from build123d import *

# Parameters (mm, degrees)
SKETCH_1_R               = 45
EXTRUDE_2_DEPTH          = 19
SKETCH_3_R               = 30
EXTRUDE_3_DEPTH          = 34
SKETCH_8_R               = 23.5
CUT_EXTRUDE_2_DEPTH      = 14
SKETCH_9_R               = 31
CUT_EXTRUDE_4_DEPTH      = 14
SKETCH_11_R              = 25
CUT_EXTRUDE_6_DEPTH      = 6
SKETCH_12_R              = 17.5
CUT_EXTRUDE_7_DEPTH      = 60
SKETCH_14_R              = 2
CUT_EXTRUDE_8_DEPTH      = 20
PATTERN_CIRCULAR_1_COUNT = 4
SKETCH_15_R              = 1.5
CUT_EXTRUDE_9_DEPTH      = 12
PATTERN_CIRCULAR_2_COUNT = 4
FILLET_1_R               = 1
SKETCH_16_R              = 4.5
CUT_EXTRUDE_10_DEPTH     = 4
PATTERN_CIRCULAR_3_COUNT = 4


with BuildPart() as part:
    # 草图1 → 凸台-拉伸2 (new body)
    with BuildSketch(Plane(origin=(0, 0, 0), x_dir=(1, 0, 0), z_dir=(0, 1, 0))):
        with Locations(Location((0, 0, 0), (0, 0, 270))):
            Circle(SKETCH_1_R)
    extrude(amount=-EXTRUDE_2_DEPTH)

    # 草图3 → 凸台-拉伸3 (add)
    with BuildSketch(Plane.XZ.offset(19)):
        with Locations(Location((0, 0, 0), (0, 0, 270))):
            Circle(SKETCH_3_R)
    extrude(amount=EXTRUDE_3_DEPTH)

    # 草图8 → 切除-拉伸2 (cut)
    with BuildSketch(Plane.XZ.offset(53)):
        with Locations(Location((0, 0, 0), (0, 0, 270))):
            Circle(SKETCH_8_R)
    extrude(amount=-CUT_EXTRUDE_2_DEPTH, mode=Mode.SUBTRACT)

    # 草图9 → 切除-拉伸4 (cut)
    with BuildSketch(Plane(origin=(0, 0, 0), x_dir=(1, 0, 0), z_dir=(0, 1, 0))):
        with Locations(Location((0, 0, 0), (0, 0, 270))):
            Circle(SKETCH_9_R)
    extrude(amount=-CUT_EXTRUDE_4_DEPTH, mode=Mode.SUBTRACT)

    # 草图11 → 切除-拉伸6 (cut)
    with BuildSketch(Plane(origin=(0, -14, 0), x_dir=(1, 0, 0), z_dir=(0, 1, 0))):
        with Locations(Location((0, 0, 0), (0, 0, 270))):
            Circle(SKETCH_11_R)
    extrude(amount=-CUT_EXTRUDE_6_DEPTH, mode=Mode.SUBTRACT)

    # 草图12 → 切除-拉伸7 (cut)
    with BuildSketch(Plane(origin=(0, -20, 0), x_dir=(1, 0, 0), z_dir=(0, 1, 0))):
        with Locations(Location((0, 0, 0), (0, 0, 270))):
            Circle(SKETCH_12_R)
    extrude(amount=-CUT_EXTRUDE_7_DEPTH, mode=Mode.SUBTRACT)

    # 草图14 → 切除-拉伸8 (cut)
    with BuildSketch(Plane(origin=(0, 0, 0), x_dir=(1, 0, 0), z_dir=(0, 1, 0))):
        with Locations(Location((0, 38, 0), (0, 0, 270))):
            Circle(SKETCH_14_R)
    cut_extrude_8 = extrude(amount=-CUT_EXTRUDE_8_DEPTH, mode=Mode.SUBTRACT)

    # 阵列(圆周)1: 切除-拉伸8 ×4 about axis
    pattern_circular_1_axis = Axis((0, 0, 0), (0, 1, 0))
    for i in range(1, PATTERN_CIRCULAR_1_COUNT):
        add(cut_extrude_8.rotate(pattern_circular_1_axis, i * 360 / PATTERN_CIRCULAR_1_COUNT), mode=Mode.SUBTRACT)

    # 草图15 → 切除-拉伸9 (cut)
    with BuildSketch(Plane.XZ.offset(53)):
        with Locations(Location((0, 27, 0), (0, 0, 270))):
            Circle(SKETCH_15_R)
    cut_extrude_9 = extrude(amount=-CUT_EXTRUDE_9_DEPTH, mode=Mode.SUBTRACT)

    # 阵列(圆周)2: 切除-拉伸9 ×4 about axis
    pattern_circular_2_axis = Axis((0, 0, 0), (0, 1, 0))
    for i in range(1, PATTERN_CIRCULAR_2_COUNT):
        add(cut_extrude_9.rotate(pattern_circular_2_axis, i * 360 / PATTERN_CIRCULAR_2_COUNT), mode=Mode.SUBTRACT)

    # 圆角1
    fillet_1_edges = [part.edges().sort_by_distance(p)[0] for p in [
        (0, 0, -45),
        (0, -19, -45),
        (0, -19, 30),
        (0, -53, 30),
    ]]
    fillet(fillet_1_edges, radius=FILLET_1_R)

    # 草图16 → 切除-拉伸10 (cut)
    with BuildSketch(Plane(origin=(0, 0, 0), x_dir=(1, 0, 0), z_dir=(0, 1, 0))):
        with Locations(Location((-38, 0, 0), (0, 0, 270))):
            Circle(SKETCH_16_R)
    cut_extrude_10 = extrude(amount=-CUT_EXTRUDE_10_DEPTH, mode=Mode.SUBTRACT)

    # 阵列(圆周)3: 切除-拉伸10 ×4 about axis
    pattern_circular_3_axis = Axis((0, 0, 0), (0, 1, 0))
    for i in range(1, PATTERN_CIRCULAR_3_COUNT):
        add(cut_extrude_10.rotate(pattern_circular_3_axis, i * 360 / PATTERN_CIRCULAR_3_COUNT), mode=Mode.SUBTRACT)


solid = part.part
The listing builds one solid part. Answer for the finished solid, in the listing's coordinates (mm). A direction names the side the tool comes from. Round coordinates to 2 decimals unless told otherwise and drop trailing zeros. Loops run counter-clockwise (first coordinate to the right, second up) from the corner with the lowest first, then second, coordinate; pieces in that order, holes last. Notation, with made-up numbers: M -7,30 L 28,30 A33 ccw 28,69 Z; hole C 34,5 d10. An arc over 180 degrees is marked long. Return JSON: item names as keys, results as strings.
Q1. Which of the six approach directions +Z, -Z, +X, -X, +Y, -Y give full straight-line access (tool end or side, diameter ignored) to faces 1 (the face through (14, -14, -21)), 2 (the face through (-27, -41, 0)), 3 (the face through (0, -11, 40))?
Results list:
{"face 1": "+Y", "face 2": "-Y", "face 3": "+Y, -Y"}
Q2. Each of these flat-tipped pins is pushed along its axis until it touches: pin 1 Ø4 at (x, z) = (-27, 0) entering from +Y; pin 2 Ø2 at (x, z) = (6, 14.5) entering from +Y; pin 3 Ø11.5 at (x, z) = (0, 38) entering from -Y; pin 4 Ø4.5 at (x, z) = (0, 38) entering from +Y. Where does it stop, or does it pass through?
Results list:
{"pin 1": "stops at y = -14", "pin 2": "passes through", "pin 3": "stops at y = -19", "pin 4": "stops at y = -4"}
Q3. Find section A-A, the plane y = -47.5. Determine the outline of the cut face in (x, z), plus the area to 3 significant figures.
Results list:
{"outline": "C 0,0 d60; hole C -27,0 d3; hole C 0,0 d47; hole C 0,-27 d3; hole C 0,27 d3; hole C 27,0 d3", "area": "1,060 mm2"}
Q4. Find the intervals of material crossed by line 1 along X through (y, z) = (-18, 1); line 2 along Y through (x, z) = (10.5, 31); line 3 along Y through (x, z) = (2, -25.5), in increasing order. Write a range as from..to.
Results list:
{"line 1": "x = -44.99..-39.73, -36.27..-24.98, 24.98..36.27, 39.73..44.99", "line 2": "y = -19..0", "line 3": "y = -53..-14"}
Q5. Find section B-B, the plane x = 0. State how many separate pieces and enclosed holes the cut face has, plus the area to 3 significant figures.
Results list:
{"separate pieces": "4", "enclosed holes": "0", "area": "994 mm2"}
Q6. The mould has two halves that part along Z. Classify faces 4 (the face through (1.32, -35.78, 29.97)), 5 (the face through (30, 0, 10)), 6 (the face through (0.98, -1.97, -42.39)): released by +Z, released by -Z, zero draft, split by the parting line, or undercut.
Results list:
{"face 4": "split by the parting line", "face 5": "zero draft", "face 6": "undercut"}
